Geometry: see drawing. Coordinates: mm, zero at the bounding-box minimum. A direction names the side the tool comes from. Coordinates: 2 decimals unless noted, no trailing zeros. Write each loop counter-clockwise with the first axis right and the second up, starting at its lowest first coordinate (ties: lowest second). Pieces come first, ordered by that corner, then holes. Notation, with made-up numbers: (82, 65.25) - (129, 65.25) arc R14 ccw to (129, 85.25) - close; hole circle Ø6 at (52.5, 3.5). An arc over 180 degrees is marked (long way). Use CSV: the item, a comma, the result in double quotes.
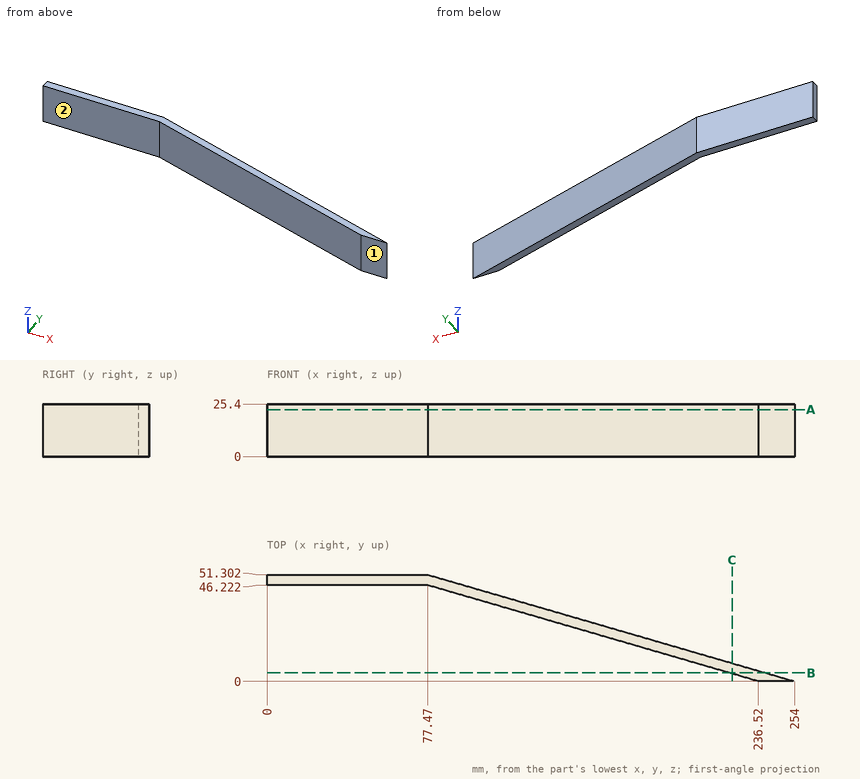
(1) Cut plane B-B on y = 4. Return loops of the section in (x, z), and give its area (3 significant figures).
Check values:
outline,"(222.76, 0) - (240.24, 0) - (240.24, 25.4) - (222.76, 25.4) - close"
area,"444 mm^2"
(2) Pin query (flat end, axial travel): pin 1 Ø6 at (x, z) = (143, 10) entering from +Y; pin 2 Ø2 at (x, z) = (32, 7) entering from -Y; pin 3 Ø1.5 at (x, z) = (182.5, 16.5) entering from -Y. Return the tip coordinate at first contact, or that it passes through.
Check values:
pin 1,"y = 33.13"
pin 2,"y = 46.22"
pin 3,"y = 15.48"
(3) Ray query, probe 1 along Y at (x, z) = (14.5, 14.75); probe 2 along Y at (x, z) = (226, 9). Return the intervals inside material, ascending. Write a range as from..to.
Check values:
probe 1,"46.22..51.3"
probe 2,"3.06..8.14"
(4) Cut plane C-C on x = 224. Return loops of the section in (y, z).
Check values:
outline,"(3.64, 0) - (8.72, 0) - (8.72, 25.4) - (3.64, 25.4) - close"
(5) Cut plane A-A on z = 22.75. Return loops of the section in (x, y), and give its area (3 significant figures).
Check values:
outline,"(0, 46.22) - (77.47, 46.22) - (236.52, 0) - (254, 0) - (77.47, 51.3) - (0, 51.3) - close"
area,"1,250 mm^2"
(6) Reachability of the marked faces 1 and 2 from +Z, -Z, +X, -X, +Y, -Y: full face, straight path, thin tool, end or side. Return the list, or none.
Check values:
face 1,"+Z, -Z, +X, -X, -Y"
face 2,"+Z, -Z, -X, -Y"
